Autodesk Inventor part; units mm, degrees
ref_plane "YZ Plane" through (0, 0, 0) normal (1, 0, 0) x (0, 1, 0)
ref_plane "XZ Plane" through (0, 0, 0) normal (0, 1, 0) x (-1, 0, 0)
ref_plane "XY Plane" through (0, 0, 0) normal (0, 0, 1) x (1, 0, 0)
sketch "Sketch1" plane through (0, 0, 0) normal (0, 1, 0) x (-1, 0, 0)
  circle A0 centre (0, 0) radius 101.6
  dimension "d0" = 203.2
extrude "Extrusion1" add sketch "Sketch1" along normal blind 6.35
sketch "Sketch3" plane through (0, 6.35, 0) normal (0, 1, 0) x (1, 0, 0)
  line L0 (0, 0) -> (87.9995, 36.4506) construction
  line L1 (0, 0) -> (95.25, 0) construction
  line L2 (87.9995, 36.4506) -> (90.4296, 30.584) construction
  point P0 (85.5695, 42.3172)
  point P1 (85.5695, 42.3172)
  dimension "d14" = 95.25
  dimension "d15" = 22.5
  dimension "d16" = 6.35
  dimension "d17" = 90
hole "Hole2" at (90.4296, 6.35, -30.584) at (85.5695, 6.35, -42.3172) direction (0, -1, 0) diameter 3.81 depth 8.8646 tip angle 118
pattern_circular "Circular Pattern2" count 8 over 360 about axis through (0, 0, 0) along (0, 1, 0) of "Hole2"
sketch "Sketch5" plane through (0, 0, 0) normal (0, -1, 0) x (1, 0, 0)
  circle A0 centre (0, 0) radius 101.6
  circle A1 centre (0, 0) radius 101.6
  circle A2 centre (0, 0) radius 98.425
  dimension "d31" = 196.85
extrude "Extrusion3" cut sketch "Sketch5" against normal blind 3.175
sketch "Sketch6" plane through (0, 6.35, 0) normal (0, 1, 0) x (1, 0, 0)
  line L0 (0, 0) -> (71.842, -71.842) construction
  line L1 (0, 0) -> (101.6, 0) construction
  line L2 (71.842, -71.842) -> (44.9013, -44.9013) construction
  circle A0 centre (44.9013, -44.9013) radius 12.7
  dimension "d39" = 101.6
  dimension "d40" = 45
  dimension "d41" = 38.1
  dimension "d42" = 25.4
extrude "Extrusion4" cut sketch "Sketch6" against normal blind 25.4
sketch "Sketch8" plane through (0, 6.35, 0) normal (0, 1, 0) x (1, 0, 0)
  circle A0 centre (44.9013, -44.9013) radius 12.7 construction
  line L0 (44.9013, -44.9013) -> (-60.1677, 60.1677) construction
  line L1 (44.9013, -44.9013) -> (193.4913, -44.9013) construction
  circle A1 centre (-60.1677, 60.1677) radius 46.99
  point P0 (0, 0)
  dimension "d64" = 148.59
  dimension "d65" = 135
  dimension "d66" = 93.98
sketch "Sketch7" plane through (0, 6.35, 0) normal (0, 1, 0) x (1, 0, 0)
  circle A0 centre (44.9013, -44.9013) radius 12.7 construction
  line L0 (44.9013, -44.9013) -> (0, 0) construction
  line L1 (44.9013, -44.9013) -> (-23.5283, 23.5283) construction
  line L2 (44.9013, -44.9013) -> (141.6753, -44.9013) construction
  circle A1 centre (-23.5283, 23.5283) radius 139.7 construction
  line L3 (-23.5283, 23.5283) -> (4.7102, 160.3445)
  line L4 (-23.5283, 23.5283) -> (116.1717, 23.5283) construction
  line L5 (-23.5283, 23.5283) -> (-160.3445, -4.7102)
  circle A2 centre (0, 0) radius 83.82 construction
  line L6 (0, 0) -> (-83.82, 0) construction
  line L7 (0, 0) -> (0, 83.82) construction
  line L8 (0, 0) -> (83.82, 0) construction
  line L9 (0, 0) -> (0, -83.82) construction
  dimension "d45" = 63.5
  dimension "d46" = 96.774
  dimension "d47" = 135
  dimension "d48" = 279.4
  dimension "d49" = 139.7
  dimension "d50" = 281.662
  dimension "d56" = 167.64
hole "Hole3" [suppressed]
extrude "Extrusion6" cut sketch "Sketch8" against normal blind 2.54
sketch "Sketch11" plane through (0, 6.35, 0) normal (0, 1, 0) x (1, 0, 0)
  circle A0 centre (44.9013, -44.9013) radius 12.7
  line L0 (44.9013, -44.9013) -> (-22.7556, 22.7556) construction
  line L1 (44.9013, -44.9013) -> (140.5826, -44.9013) construction
  circle A1 centre (0, 0) radius 86.36 construction
  arc A2 (-96.8278, 30.7722) -> (-30.7722, 96.8278) centre (0, 0) ccw
  line L2 (-22.7556, 22.7556) -> (-22.556, -104.2442) construction
  line L3 (-22.7556, 22.7556) -> (-167.6337, -24.8282)
  line L4 (-22.7556, 22.7556) -> (-15.9096, -104.0597) construction
  circle A3 centre (-22.7556, 22.7556) radius 127 construction
  line L5 (-22.7556, 22.7556) -> (-29.2029, -104.0806) construction
  line L6 (-22.7556, 22.7556) -> (-145.323, -10.5045) construction
  line L7 (-22.7556, 22.7556) -> (-141.175, -23.134) construction
  circle A4 centre (-145.323, -10.5045) radius 64.77 construction
  circle A5 centre (-141.175, -23.134) radius 64.77 construction
  circle A6 centre (-29.2029, -104.0806) radius 66.04 construction
  circle A7 centre (-15.9096, -104.0597) radius 66.04 construction
  point P0 (-85.2605, 13.7369)
  point P1 (-77.9464, -37.1807)
  point P2 (43.2653, -74.7406)
  point P3 (-69.2646, -51.5797)
  point P4 (-13.7369, 85.2605)
  point P5 (37.1807, 77.9464)
  point P6 (74.7406, -43.2653)
  point P7 (51.5797, 69.2646)
  dimension "d117" = 129.54
  dimension "d118" = 132.08
  dimension "d109" = 135
  dimension "d110" = 95.6813
  dimension "d111" = 172.72
  dimension "d112" = 44.91
  dimension "d113" = 116.818
  dimension "d114" = 3
  dimension "d115" = 254
  dimension "d116" = 3
hole "Hole5" at (-85.2605, 6.35, -13.7369) at (-77.9464, 6.35, 37.1807) at (43.2653, 6.35, 74.7406) at (-69.2646, 6.35, 51.5797) at (37.1807, 6.35, -77.9464) at (51.5797, 6.35, -69.2646) at (-13.7369, 6.35, -85.2605) at (74.7406, 6.35, 43.2653) direction (0, -1, 0) diameter 6.7564 depth 25.4 tip angle 118
properties part number "4K sheild top" material "Copper"
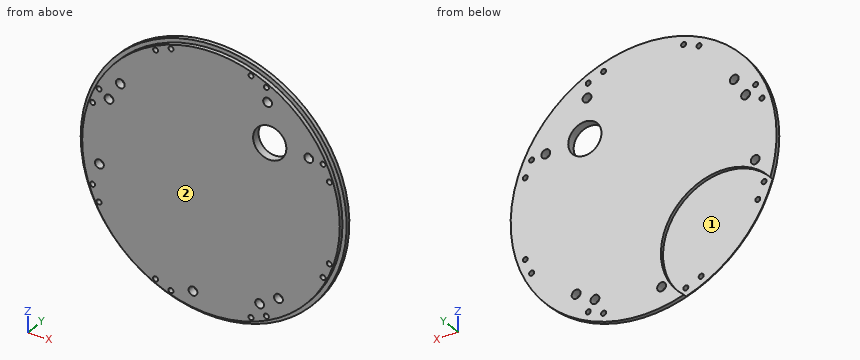
Source: CAD feature listing. Evaluate the final solid. Frame: model axes, mm. Face numbers are marked on the shaded views. Give positions to 0.01 mm unless a question says otherwise; leave off trailing zeros. Write each loop counter-clockwise with the first axis right and the second up, starting at its lowest first coordinate (ties: lowest second). Pieces come first, ordered by that corner, then holes. Notation, with made-up numbers: M 20.25,69 L 69.25,69 A23 ccw 69.25,98 Z; hole C -9,27.25 d10. An arc over 180 degrees is marked long. Return JSON: item names as keys, results as strings. Group by question number.
1) Cut plane B-B, the plane z = 0. Output: boundary loops of the cut face in (x, y) (3 decimals), then the cut area to 3 significant figures.
2) Ray query, L1, parallel to X at y = 2.5, z = -91.5; L2, parallel to X at y = 5.75, z = 46; L3, parallel to Z at x = 41, y = 3. Return the intervals inside material, ascending.
3) Cut plane C-C, the plane x = 0. Output: boundary loops of the cut face in (y, z) (3 decimals), then the cut area to 3 significant figures.
4) Cut plane D-D, the plane x = -52. Output: boundary loops of the cut face in (y, z) (3 decimals).
5) Draft query along Z for the marked faces 1 and 2. Return one class per face: released by +Z, released by -Z, zero draft, split by the parting line, or undercut.
6) Cut plane A-A, the plane y = 1.5. Give the number of separate pieces and of enclosed holes in the cut face, then the cut area to 3 significant figures.
7) First-contact query: pin 1 Ø2.5 at (x, z) = (90.43, -30.58) entering from +Y; pin 2 Ø5 at (x, z) = (-30.58, -90.43) entering from +Y; pin 3 Ø3 at (y, z) = (2, -29) entering from +X; pin 4 Ø1.5 at (x, y) = (50, 3) entering from -Z. Flat tips, straight axial feed; report the tip coordinate or a pass-through.
Data:
{
 "1": {"outline": "M -101.6,3.175 L -98.425,3.175 L -98.425,0 L 98.425,0 L 98.425,3.175 L 101.6,3.175 L 101.6,6.35 L -101.6,6.35 Z", "area": "1,270 mm²"},
 "2": {"L1": "x = -36.27 to -32.16, -29.01 to 29.01, 32.16 to 36.27", "L2": "x = -90.59 to 32.25, 57.55 to 72.76, 76.72 to 90.59", "L3": "z = -89.48 to -86.95, -84.19 to 32.82, 56.99 to 72.23, 77.25 to 84.19, 86.95 to 89.48"},
 "3": {"outline": "M 0,-98.425 L 3.175,-98.425 L 3.175,-101.6 L 6.35,-101.6 L 6.35,101.6 L 3.175,101.6 L 3.175,98.425 L 0,98.425 Z", "area": "1,270 mm²"},
 "4": {"outline": "M 0,-83.567 L 3.175,-83.567 L 3.175,-87.284 L 3.81,-87.284 L 3.81,-13.893 L 6.35,-13.893 L 6.35,87.284 L 3.175,87.284 L 3.175,83.567 L 0,83.567 Z"},
 "5": {"face 1": "undercut", "face 2": "zero draft"},
 "6": {"separate pieces": "1", "enclosed holes": "25", "area": "29,500 mm²"},
 "7": {"pin 1": "passes through", "pin 2": "stops at y = 3.81", "pin 3": "stops at x = 97.65", "pin 4": "stops at z = -88.85"}
}
